Part model, mm, in its own coordinate system. Round coordinates to 2 decimals unless told otherwise and drop trailing zeros. Loops run counter-clockwise (first coordinate to the right, second up) from the corner with the lowest first, then second, coordinate; pieces in that order, holes last.
from build123d import *

# Parameters (mm, degrees)
SKETCH_1_W          = 15
SKETCH_1_H          = 15
SKETCH_1_W_2        = 12
SKETCH_1_H_2        = 12
EXTRUDE_1_DEPTH     = 600
SKETCH_3_R          = 2.7
CUT_EXTRUDE_2_DEPTH = 25
SKETCH_4_R          = 2.7
CUT_EXTRUDE_3_DEPTH = 20
SKETCH_6_R          = 2.7
CUT_EXTRUDE_5_DEPTH = 30
SKETCH_7_R          = 5
CUT_EXTRUDE_6_DEPTH = 10
SKETCH_8_R          = 5
CUT_EXTRUDE_7_DEPTH = 10
SKETCH_9_R          = 5
CUT_EXTRUDE_8_DEPTH = 10


with BuildPart() as part:
    # ｽｹｯﾁ1 → ﾎﾞｽ - 押し出し1 (new body)
    with BuildSketch(Plane.XY):
        Rectangle(SKETCH_1_W, SKETCH_1_H)
        Rectangle(SKETCH_1_W_2, SKETCH_1_H_2, mode=Mode.SUBTRACT)
    extrude(amount=EXTRUDE_1_DEPTH)

    # ｽｹｯﾁ3 → ｶｯﾄ - 押し出し2 (cut)
    with BuildSketch(Plane(origin=(0, 7.5, 0), x_dir=(1, 0, 0), z_dir=(0, 1, 0))):
        with Locations((0, -7.5)):
            Circle(SKETCH_3_R)
        with Locations((0, -592.5)):
            Circle(SKETCH_3_R)
        with Locations((0, -233.5)):
            Circle(SKETCH_3_R)
        with Locations((0, -366.5)):
            Circle(SKETCH_3_R)
    extrude(amount=-CUT_EXTRUDE_2_DEPTH, mode=Mode.SUBTRACT)

    # ｽｹｯﾁ4 → ｶｯﾄ - 押し出し3 (cut)
    with BuildSketch(Plane(origin=(7.5, 0, 0), x_dir=(0, 0, -1), z_dir=(1, 0, 0))):
        with Locations((-536, 0)):
            Circle(SKETCH_4_R)
        with Locations((-501, 0)):
            Circle(SKETCH_4_R)
        with Locations((-99, 0)):
            Circle(SKETCH_4_R)
        with Locations((-64, 0)):
            Circle(SKETCH_4_R)
        with Locations((-468, 0)):
            Circle(SKETCH_4_R)
        with Locations((-550, 0)):
            Circle(SKETCH_4_R)
        with Locations((-405, 0)):
            Circle(SKETCH_4_R)
        with Locations((-195, 0)):
            Circle(SKETCH_4_R)
        with Locations((-50, 0)):
            Circle(SKETCH_4_R)
        with Locations((-132, 0)):
            Circle(SKETCH_4_R)
    extrude(amount=-CUT_EXTRUDE_3_DEPTH, mode=Mode.SUBTRACT)

    # ｽｹｯﾁ6 → ｶｯﾄ - 押し出し5 (cut)
    with BuildSketch(Plane(origin=(0, 7.5, 0), x_dir=(1, 0, 0), z_dir=(0, 1, 0))):
        with Locations((0, -435)):
            Circle(SKETCH_6_R)
        with Locations((0, -415)):
            Circle(SKETCH_6_R)
        with Locations((0, -165)):
            Circle(SKETCH_6_R)
        with Locations((0, -185)):
            Circle(SKETCH_6_R)
        with Locations((0, -347.5)):
            Circle(SKETCH_6_R)
        with Locations((0, -252.5)):
            Circle(SKETCH_6_R)
    extrude(amount=-CUT_EXTRUDE_5_DEPTH, mode=Mode.SUBTRACT)

    # ｽｹｯﾁ7 → ｶｯﾄ - 押し出し6 (cut)
    with BuildSketch(Plane(origin=(0, 7.5, 0), x_dir=(1, 0, 0), z_dir=(0, 1, 0))):
        with Locations((0, -592.5)):
            Circle(SKETCH_7_R)
        with Locations((0, -7.5)):
            Circle(SKETCH_7_R)
        with Locations((0, -185)):
            Circle(SKETCH_7_R)
        with Locations((0, -165)):
            Circle(SKETCH_7_R)
        with Locations((0, -435)):
            Circle(SKETCH_7_R)
        with Locations((0, -415)):
            Circle(SKETCH_7_R)
        with Locations((0, -366.5)):
            Circle(SKETCH_7_R)
        with Locations((0, -233.5)):
            Circle(SKETCH_7_R)
        with Locations((0, -252.5)):
            Circle(SKETCH_7_R)
        with Locations((0, -347.5)):
            Circle(SKETCH_7_R)
    extrude(amount=-CUT_EXTRUDE_6_DEPTH, mode=Mode.SUBTRACT)

    # ｽｹｯﾁ8 → ｶｯﾄ - 押し出し7 (cut)
    with BuildSketch(Plane(origin=(7.5, 0, 0), x_dir=(0, 0, -1), z_dir=(1, 0, 0))):
        with Locations((-64, 0)):
            Circle(SKETCH_8_R)
        with Locations((-99, 0)):
            Circle(SKETCH_8_R)
        with Locations((-536, 0)):
            Circle(SKETCH_8_R)
        with Locations((-501, 0)):
            Circle(SKETCH_8_R)
    extrude(amount=-CUT_EXTRUDE_7_DEPTH, mode=Mode.SUBTRACT)

    # ｽｹｯﾁ9 → ｶｯﾄ - 押し出し8 (cut)
    with BuildSketch(Plane.ZY.offset(7.5)):
        with Locations((468, 0)):
            Circle(SKETCH_9_R)
        with Locations((405, 0)):
            Circle(SKETCH_9_R)
        with Locations((550, 0)):
            Circle(SKETCH_9_R)
        with Locations((195, 0)):
            Circle(SKETCH_9_R)
        with Locations((50, 0)):
            Circle(SKETCH_9_R)
        with Locations((132, 0)):
            Circle(SKETCH_9_R)
    extrude(amount=-CUT_EXTRUDE_8_DEPTH, mode=Mode.SUBTRACT)


solid = part.part
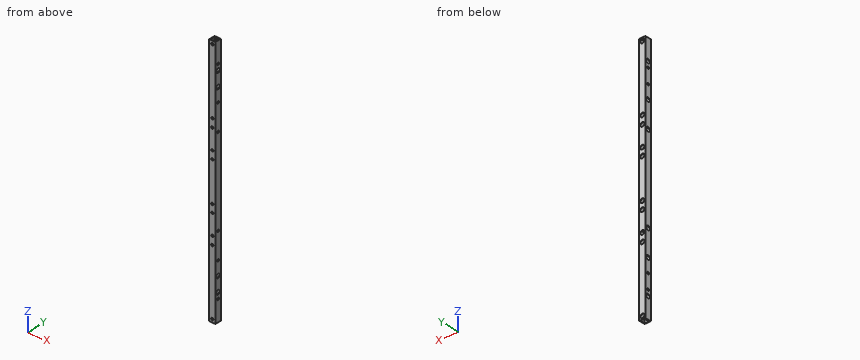
1) Wall check: line 1 along Y through (x, z) = (-2.5, 95); line 2 along Y through (x, z) = (-6.35, 64). Give the ranges that are in metal, low to high.
Values:
line 1: y = -7.5 to -6, 6 to 7.5
line 2: y = -7.5 to -2.7, 2.7 to 7.5
2) Slice it at B-B, the plane y = 0. Give the number of separate pieces and of enclosed holes in the cut face, then the cut area to 3 significant figures.
Values:
separate pieces: 22
enclosed holes: 0
area: 1,570 mm2
3) Slice it at A-A, the plane z = 311. Give the cut face in (x, y), then the cut area to 3 significant figures.
Values:
outline: (-7.5, -7.5) - (7.5, -7.5) - (7.5, 7.5) - (-7.5, 7.5) - close; hole (-6, -6) - (6, -6) - (6, 6) - (-6, 6) - close
area: 81.0 mm2
4) Drop flat-ended pins along their axis: pin 1 Ø7 at (y, z) = (0, 99) entering from +X; pin 2 Ø7 at (x, z) = (0, 252.5) entering from +Y; pin 3 Ø8 at (x, z) = (0, 366.5) entering from -Y; pin 4 Ø6 at (y, z) = (0, 468) entering from -X. Give the stop position or say it passes through.
Values:
pin 1: stops at x = -6
pin 2: stops at y = -6
pin 3: stops at y = -7.5
pin 4: stops at x = 6
